```python
from build123d import *

# Parameters (mm, degrees)
SKETCH1_R           = 2.5
BOSS_EXTRUDE2_DEPTH = 3


with BuildPart() as part:
    # Sketch1 → Boss-Extrude2 (new body)
    with BuildSketch(Plane(origin=(0, 0, 0), x_dir=(1, 0, 0), z_dir=(0, 1, 0))):
        with BuildLine():
            Line((0, 19.583928173), (0, 53.583928173))
            ThreePointArc((0, 53.583928173), (0.878679656, 55.705248517), (3, 56.583928173))
            Line((3, 56.583928173), (75, 56.583928173))
            ThreePointArc((75, 56.583928173), (78.535533906, 55.119462079), (80, 51.583928173))
            Line((80, 51.583928173), (80, -0.416071827))
            ThreePointArc((80, -0.416071827), (79.121320344, -2.537392171), (77, -3.416071827))
            Line((77, -3.416071827), (23, -3.416071827))
            ThreePointArc((23, -3.416071827), (20.878679656, -2.537392171), (20, -0.416071827))
            Line((20, -0.416071827), (20, 16.583928173))
            Line((20, 16.583928173), (3, 16.583928173))
            ThreePointArc((3, 16.583928173), (0.878679656, 17.462607829), (0, 19.583928173))
        make_face()
        with Locations((10, 26.583928173)):
            Circle(SKETCH1_R, mode=Mode.SUBTRACT)
        with Locations((40, 6.583928173)):
            Circle(SKETCH1_R, mode=Mode.SUBTRACT)
        with Locations((70, 6.583928173)):
            Circle(SKETCH1_R, mode=Mode.SUBTRACT)
        with Locations((10, 46.583928173)):
            Circle(SKETCH1_R, mode=Mode.SUBTRACT)
        with BuildLine():
            Line((40, 39.083928173), (70, 39.083928173))
            ThreePointArc((70, 39.083928173), (72.5, 36.583928173), (70, 34.083928173))
            Line((70, 34.083928173), (40, 34.083928173))
            ThreePointArc((40, 34.083928173), (37.5, 36.583928173), (40, 39.083928173))
        make_face(mode=Mode.SUBTRACT)
    extrude(amount=BOSS_EXTRUDE2_DEPTH)


solid = part.part
```
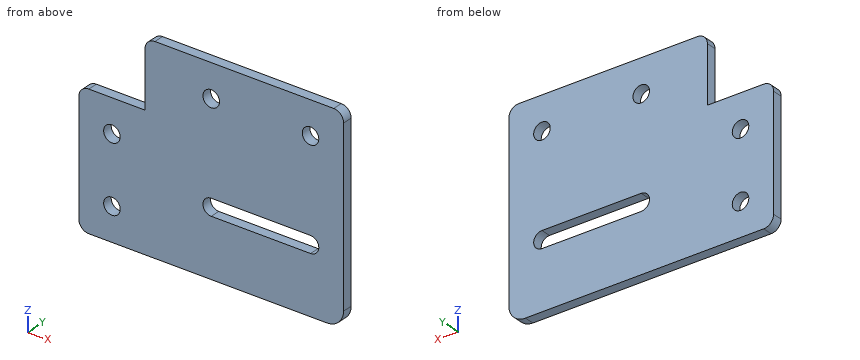
CAD build for the part. Positions are in the model's coordinates, mm. Round coordinates to 2 decimals unless told otherwise and drop trailing zeros. Order: outer loops, then holes, each group sorted by start corner. A loop starts at its lowest first (then second) coordinate and runs counter-clockwise, first axis right, second up. Notation, with made-up numbers: (-29, 2.25) - (12, 2.25) arc R28 ccw to (12, 40.25) - close; hole circle Ø6 at (-24.5, 59.5). An arc over 180 degrees is marked (long way). Use CSV: the item, a comma, the result in double quotes. Start each with the question number.
1) Saw through at A-A (x = 47). List the corners of the cut face in (y, z).
2) Saw through at D-D (y = 0.8). List the corners of the cut face in (x, z).
3) Saw through at C-C (z = -36). List the corners of the cut face in (x, y).
4) Saw through at B-B (x = 10). List the corners of the cut face in (y, z), and give its area (3 significant figures).
5) Pin check, flat tips, straight feed: pin 1 Ø4 at (x, z) = (10, -26.58) entering from -Y; pin 2 Ø1.5 at (x, y) = (15.5, 2) entering from +Z; pin 3 Ø0.9 at (y, z) = (1.5, -7.5) entering from -X. Stop position of each tip, or through.
6) Wall check: L1, parallel to Z at x = 40, y = 1.6; L2, parallel to Z at x = 62, y = 0.5; L3, parallel to Z at x = 10, y = 1.1. Give the ranges that are in metal, low to high. Write a range as [from, to].
Values follow:
1,outline,"(0, -56.58) - (3, -56.58) - (3, -39.08) - (0, -39.08) - close; (0, -34.08) - (3, -34.08) - (3, 3.42) - (0, 3.42) - close"
2,outline,"(0, -53.58) arc R3 ccw to (3, -56.58) - (75, -56.58) arc R5 ccw to (80, -51.58) - (80, 0.42) arc R3 ccw to (77, 3.42) - (23, 3.42) arc R3 ccw to (20, 0.42) - (20, -16.58) - (3, -16.58) arc R3 ccw to (0, -19.58) - close; hole circle Ø5 at (10, -46.58); hole circle Ø5 at (10, -26.58); hole circle Ø5 at (40, -6.58); hole (40, -39.08) - (70, -39.08) arc R2.5 ccw to (70, -34.08) - (40, -34.08) arc R2.5 ccw to start; hole circle Ø5 at (70, -6.58)"
3,outline,"(0, 0) - (37.57, 0) - (37.57, 3) - (0, 3) - close; (72.43, 0) - (80, 0) - (80, 3) - (72.43, 3) - close"
4,outline,"(0, -56.58) - (3, -56.58) - (3, -49.08) - (0, -49.08) - close; (0, -44.08) - (3, -44.08) - (3, -29.08) - (0, -29.08) - close; (0, -24.08) - (3, -24.08) - (3, -16.58) - (0, -16.58) - close"
4,area,"90.0 mm2"
5,pin 1,"passes through"
5,pin 2,"stops at z = -16.58"
5,pin 3,"stops at x = 20"
6,L1,"z = [-56.58, -39.08], [-34.08, -9.08], [-4.08, 3.42]"
6,L2,"z = [-56.58, -39.08], [-34.08, 3.42]"
6,L3,"z = [-56.58, -49.08], [-44.08, -29.08], [-24.08, -16.58]"
